Autodesk Inventor part; units mm, degrees
ref_plane "YZ Plane" through (0, 0, 0) normal (1, 0, 0) x (0, 1, 0)
ref_plane "XZ Plane" through (0, 0, 0) normal (0, 1, 0) x (-1, 0, 0)
ref_plane "XY Plane" through (0, 0, 0) normal (0, 0, 1) x (1, 0, 0)
sketch "Esquisse1" plane through (0, 0, 0) normal (0, 1, 0) x (-1, 0, 0)
  circle A0 centre (0, 0) radius 25 construction
  line L0 (-25, 0) -> (25, 0) construction
  arc A1 (-75, -80.7775) -> (-75, 80.7775) centre (-25, 0) ccw construction
  arc A2 (75, 80.7775) -> (75, -80.7775) centre (25, 0) ccw construction
  line L1 (0, 25) -> (0, 0) construction
  line L2 (-75, 80.7775) -> (75, 80.7775)
  line L3 (-75, -80.7775) -> (75, -80.7775)
  arc A3 (75, -80.7775) -> (75, 80.7775) centre (25, 0) ccw
  arc A4 (-75, 80.7775) -> (-75, -80.7775) centre (-25, 0) ccw
  dimension "d0" = 50
  dimension "d1" = 190
  dimension "d2" = 150
extrude "Extrusion1" add sketch "Esquisse1" along normal blind 4
sketch "Esquisse16" plane through (0, 0, 0) normal (0, -1, 0) x (1, 0, 0)
  line L0 (-70, 70) -> (70, 70) construction
  line L1 (70, 70) -> (70, -70) construction
  line L2 (70, -70) -> (-70, -70) construction
  line L3 (-70, -70) -> (-70, 70) construction
  circle A0 centre (70, 70) radius 3
  circle A1 centre (-70, 70) radius 3
  circle A2 centre (-70, -70) radius 3
  circle A3 centre (70, -70) radius 3
  point P0 (0, 0)
  dimension "d146" = 140
  dimension "d147" = 140
  dimension "d148" = 6
  dimension "d149" = 6
  dimension "d150" = 6
  dimension "d151" = 6
  dimension "d152" = 70
  dimension "d153" = 70
extrude "Extrusion13" cut sketch "Esquisse16" against normal through all
sketch "Esquisse18" plane through (0, 0, 0) normal (0, -1, 0) x (1, 0, 0)
  line L0 (-90, 40) -> (90, 40) construction
  line L1 (90, 40) -> (90, -40) construction
  line L2 (90, -40) -> (-90, -40) construction
  line L3 (-90, -40) -> (-90, 40) construction
  circle A0 centre (-90, 40) radius 12.5
  circle A1 centre (90, 40) radius 12.5
  circle A2 centre (90, -40) radius 12.5
  circle A3 centre (-90, -40) radius 12.5
  point P0 (0, 0)
  dimension "d170" = 180
  dimension "d171" = 90
  dimension "d172" = 80
  dimension "d173" = 40
  dimension "d174" = 25
  dimension "d175" = 25
  dimension "d176" = 25
  dimension "d177" = 25
extrude "Extrusion15" cut sketch "Esquisse18" against normal through all
properties part number "base"
Geometry: final body of the model. Coordinates: model frame, mm. Round coordinates to 2 decimals unless told otherwise and drop trailing zeros. Write each loop counter-clockwise with the first axis right and the second up, starting at its lowest first coordinate (ties: lowest second). Pieces come first, ordered by that corner, then holes. Notation, with made-up numbers: M 39,88.25 L 51,88.25 A10 cw 51,104.25 Z; hole C -28.75,45 d1. An arc over 180 degrees is marked long. Answer in a Markdown table with one row per item. Add a question column.
(1) Draft query along X for faces 1 (the face through (-119.99, 1.97, 1.35)), 2 (the face through (-72.4, 2, 68.2)), 3 (the face through (2, 4, 1)). Return one class per face: pulls with the +X half, pulls with the -X half, needs draft (parallel to the pull), parting line crosses it, or undercut.
(2) Cut plane C-C, the plane z = 30. Return the cut outline in (x, y), then the cut area to 3 significant figures.
(3) Cut plane A-A, the plane y = 3. Give the number of separate pieces and of enclosed holes in the cut face, then the cut area to 3 significant figures.
(4) Ray query, L1, parallel to Z at x = -70, y = 1.05; L2, parallel to X at y = 2.3, z = 37; L3, parallel to Z at x = -99.5, y = 1.3. Return the intervals inside material, ascending.
(5) Cut plane B-B, the plane x = 70. Return the cut outline in (y, z), then the cut area to 3 significant figures.
(6) Contact query for flat-ended pins moving along their axis: pin 1 (1.5 mm diameter, centred on y = 3.5, z = -25.5, fed in from -X); pin 2 (2 mm diameter, centred on y = 1, z = 20.5, fed in from -X); pin 3 (2 mm diameter, centred on y = 2, z = 35, fed in from -X). Output: stop coordinate, or through.
Established:
| question | item | result |
|---|---|---|
| 1 | face 1 | pulls with the -X half |
| 1 | face 2 | undercut |
| 1 | face 3 | needs draft |
| 2 | outline | M -115.14,0 L -97.5,0 L -97.5,4 L -115.14,4 Z; M -82.5,0 L 82.5,0 L 82.5,4 L -82.5,4 Z; M 97.5,0 L 115.14,0 L 115.14,4 L 97.5,4 Z |
| 2 | area | 801 mm² |
| 3 | separate pieces | 1 |
| 3 | enclosed holes | 8 |
| 3 | area | 32,400 mm² |
| 4 | L1 | -80.78 to -73, -67 to 67, 73 to 80.78 |
| 4 | L2 | -112.5 to -102.13, -77.87 to 77.87, 102.13 to 112.5 |
| 4 | L3 | -58.95 to -48.12, -31.88 to 31.88, 48.12 to 58.95 |
| 5 | outline | M 0,-80.78 L 4,-80.78 L 4,-73 L 0,-73 Z; M 0,-67 L 4,-67 L 4,67 L 0,67 Z; M 0,73 L 4,73 L 4,80.78 L 0,80.78 Z |
| 5 | area | 598 mm² |
| 6 | pin 1 | x = -116.72 |
| 6 | pin 2 | x = -117.98 |
| 6 | pin 3 | x = -113.71 |
